The model under review builds one solid part; all positions refer to its coordinate system, in mm. A direction names the side the tool comes from. Give positions to 0.01 mm unless a question says otherwise; leave off trailing zeros. Order: outer loops, then holes, each group sorted by start corner. A loop starts at its lowest first (then second) coordinate and runs counter-clockwise, first axis right, second up. Notation, with made-up numbers: (74.5, -28) - (122.5, -28) arc R25 cw to (122.5, -8) - close; hole circle Ø11 at (-17.5, 85). An arc over 180 degrees is marked (long way). Use CSV: the item, a comma, the result in double quotes. Start each with the question number.
1. Machinability: for faces 1 (the flat face through (-4, 3, 0)), 2 (the flat face through (-4, 5, 5)), which of the approach directions +Z, -Z, +X, -X, +Y, -Y give a long, thin tool a straight path to every point of the face, cutting with its end or side? Answer none if there is none.
2. For pin 1 (3 mm diameter, centred on x = -280, z = 170, fed in from -Y); pin 2 (2 mm diameter, centred on x = 119.5, z = 151, fed in from +Y), all flat-tipped, find the tip position at first contact; note any pin that passes through.
3. Take a section at A-A, the plane x = -204. State the section outline as (y, z) points, then the cut area to 3 significant figures.
4. To check wall thickness, follow line 1 (X direction, y = -205.8, z = 170); line 2 (Z direction, x = 300, y = -204.55); line 3 (Z direction, x = 206, y = -59). State the ranges of each line that lie inside material, in increasing order. Write a range as [from, to].
5. Take a section at B-B, the plane y = -102.5. State the section outline as (x, z) points, then the cut area to 3 significant figures.
6. Take a section at C-C, the plane z = 96.5. State the section outline as (x, y) points.
```python
from build123d import *

# Parameters (mm, degrees)
F0_W      = 620
F0_H      = 415
F1_DEPTH  = 5
F2_W      = 620
F2_H      = 5
F3_DEPTH  = 175
F5_D      = 5
F7_D      = 5
F9_D      = 5
F11_D     = 5
F13_D     = 5
F15_D     = 5
F17_D     = 5
F19_D     = 5
F21_D     = 5
F21_DEPTH = 11


with BuildPart() as f1:
    # F0 (on Top) → F1 (new body)
    with BuildSketch(Plane.XY):
        Rectangle(F0_W, F0_H)
    extrude(amount=F1_DEPTH)

    # F2 (on face) → F3 (join)
    with BuildSketch(Plane.XY.offset(5)):
        with Locations((0, -205)):
            Rectangle(F2_W, F2_H)
    extrude(amount=F3_DEPTH)

    # F5 (through all)
    with Locations(Plane.XZ.offset(207.5)):
        with Locations((300, 170)):
            Hole(F5_D / 2)

    # F7 (through all)
    with Locations(Plane.XZ.offset(207.5)):
        with Locations((300, 150)):
            Hole(F7_D / 2)

    # F9 (through all)
    with Locations(Plane.XZ.offset(207.5)):
        with Locations((-280, 170)):
            Hole(F9_D / 2)

    # F11 (through all)
    with Locations(Plane.XZ.offset(207.5)):
        with Locations((-280, 150)):
            Hole(F11_D / 2)

    # F13 (through all)
    with Locations(Plane.XZ.offset(207.5)):
        with Locations((-305, 175)):
            Hole(F13_D / 2)

    # F15 (through all)
    with Locations(Plane.XZ.offset(207.5)):
        with Locations((-305, 10)):
            Hole(F15_D / 2)

    # F17 (through all)
    with Locations(Plane(origin=(0, 0, 0), x_dir=(1, 0, 0), z_dir=(0, 0, -1))):
        with Locations((290, 195)):
            Hole(F17_D / 2)

    # F19 (through all)
    with Locations(Plane(origin=(0, 0, 0), x_dir=(1, 0, 0), z_dir=(0, 0, -1))):
        with Locations((-290, 195)):
            Hole(F19_D / 2)

    # F21
    with Locations(Plane.XZ.offset(207.5)):
        with Locations((285, 25)):
            Hole(F21_D / 2, depth=F21_DEPTH)


solid = f1.part
```
Determined:
1,face 1,"-Z, +X, -X, +Y, -Y"
1,face 2,"+Z, +X, -X, +Y"
2,pin 1,"passes through"
2,pin 2,"stops at y = -202.5"
3,outline,"(-207.5, 0) - (207.5, 0) - (207.5, 5) - (-202.5, 5) - (-202.5, 180) - (-207.5, 180) - close"
3,area,"2,950 mm²"
4,line 1,"x = [-310, -282.5], [-277.5, 297.5], [302.5, 310]"
4,line 2,"z = [0, 147.5], [152.5, 167.5], [172.5, 180]"
4,line 3,"z = [0, 5]"
5,outline,"(-310, 0) - (310, 0) - (310, 5) - (-310, 5) - close"
5,area,"3,100 mm²"
6,outline,"(-310, -207.5) - (310, -207.5) - (310, -202.5) - (-310, -202.5) - close"
